```python
from build123d import *

# Parameters (mm, degrees)
SKETCH1_R           = 2.5
BOSS_EXTRUDE1_DEPTH = 2.6


with BuildPart() as part:
    # Sketch1 → Boss-Extrude1 (new, symmetric)
    with BuildSketch(Plane(origin=(0, 0, 0), x_dir=(1, 0, 0), z_dir=(0, 1, 0))):
        Polygon((5.773502692, 0), (2.886751346, 5), (-2.886751346, 5), (-5.773502692, 0), (-2.886751346, -5), (2.886751346, -5), align=None)
        with Locations(Location((0, 0, 0), (0, 0, 270))):
            Circle(SKETCH1_R, mode=Mode.SUBTRACT)
    extrude(amount=BOSS_EXTRUDE1_DEPTH, both=True)

    # Sketch3 → Cut-Revolve2 (revolve, cut)
    with BuildSketch(Plane(origin=(0, 0, 0), x_dir=(0, 0, -1), z_dir=(1, 0, 0))):
        Polygon((4.133974596, 3.1), (5.866025404, 2.1), (6.366025404, 2.966025404), (4.633974596, 3.966025404), align=None)
    cut_revolve2 = revolve(axis=Axis((0, -2.6, 0), (0, 1, 0)), mode=Mode.SUBTRACT)

    # Mirror1: Cut-Revolve2 across plane
    add(cut_revolve2.mirror(Plane.ZX), mode=Mode.SUBTRACT)


solid = part.part
```
Input: part model. Units: mm. Frame: model coordinates. Give positions to 0.01 mm unless a question says otherwise; leave off trailing zeros. Order: outer loops, then holes, each group sorted by start corner. A loop starts at its lowest first (then second) coordinate and runs counter-clockwise, first axis right, second up.
1. Section A-A on y = 1.65. Return the cut outline in (x, z).
Derived:
outline: (-5.77, 0) - (-2.89, -5) - (2.89, -5) - (5.77, 0) - (2.89, 5) - (-2.89, 5) - close; hole circle Ø5 at (0, 0)
2. Pin query (flat end, axial travel): pin 1 (1 mm diameter, centred on x = -3.5, y = 1.5, fed in from +Z); pin 2 (1 mm diameter, centred on y = -1.5, z = 2.5, fed in from +X). Return the tip coordinate at first contact, or that it passes through.
Derived:
pin 1: stops at z = 4.8
pin 2: stops at x = 4.62
3. Mould query, pull axis X, two halves, no side actions, for faces 1 (the cylindrical face through (-2.44, -0.04, -0.54)), 2 (the conical face through (2.58, 2.49, 4.5)), 3 (the conical face through (-2.58, -2.49, -4.5)). Classes: released by +X, released by -X, zero draft, split by the parting line, or undercut.
Derived:
face 1: undercut
face 2: released by +X
face 3: released by -X
4. Section B-B on y = 2.3. Return the cut outline in (x, z), and give its area (3 significant figures).
Derived:
outline: (-5.5, -0.48) - (-3.16, -4.52) arc R5.52 ccw to (-2.34, -5) - (2.34, -5) arc R5.52 ccw to (3.16, -4.52) - (5.5, -0.48) arc R5.52 ccw to (5.5, 0.48) - (3.16, 4.52) arc R5.52 ccw to (2.34, 5) - (-2.34, 5) arc R5.52 ccw to (-3.16, 4.52) - (-5.5, 0.48) arc R5.52 ccw to start; hole circle Ø5 at (0, 0)
area: 66.3 mm2
5. Material intervals for L1, parallel to Z at x = 1.25, y = 1.05; L2, parallel to Z at x = -0.5, y = -2.05; L3, parallel to X at y = -2, z = -0.75, sorted ascending.
Derived:
L1: z = -5 to -2.17, 2.17 to 5
L2: z = -5 to -2.45, 2.45 to 5
L3: x = -5.34 to -2.38, 2.38 to 5.34
